The figure shows three views and two pictorial views of one solid part (mm, origin at its lowest corner). Answer the questions. A direction names the side the tool comes from. Coordinates: 2 decimals unless noted, no trailing zeros. Order: outer loops, then holes, each group sorted by start corner. A loop starts at its lowest first (then second) coordinate and runs counter-clockwise, first axis right, second up.
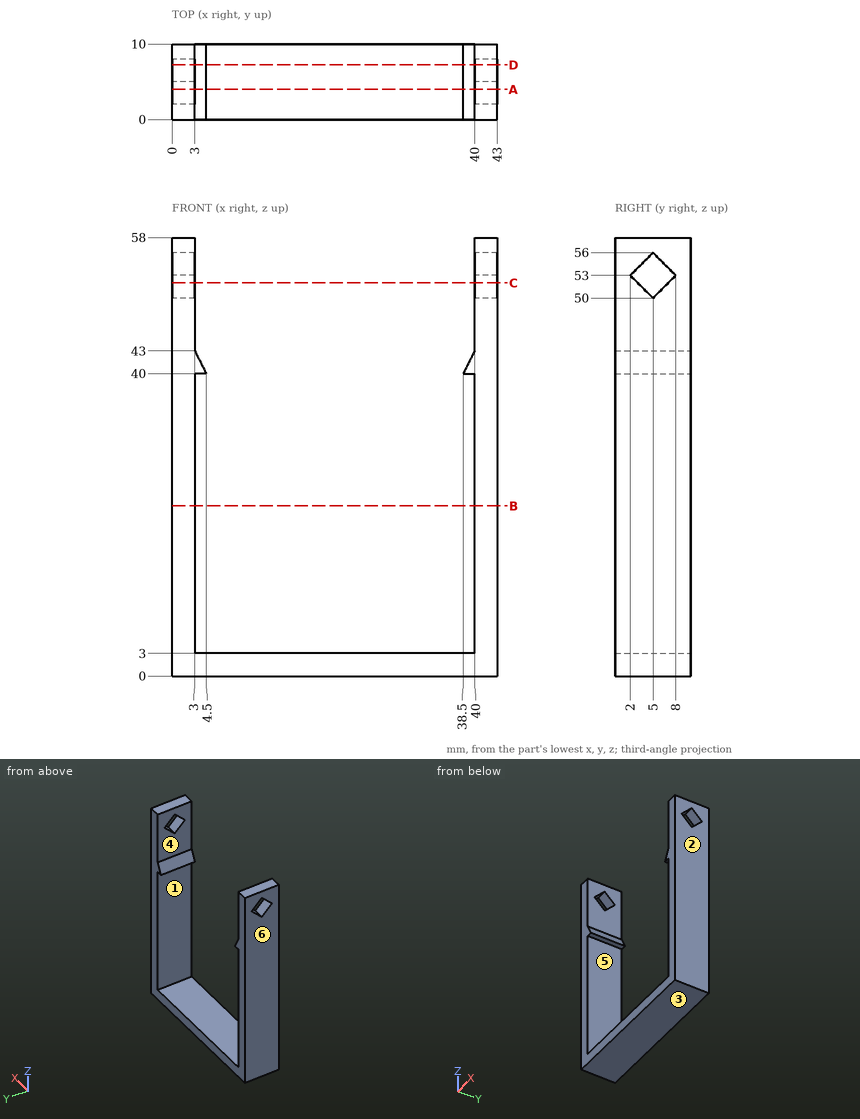
1) A cutting plane is placed at B-B, the plane z = 22.5. Write down the section's boundary in (x, y).
2) This flat-tipped pin is pushed along its axis until it touches: P1, Ø2, axis at x = 6, y = 2.5, coming from the +Z side. Where does it stop, or does it pass through?
3) For the marked faces 4, 5 and 6, determine the directions among +Z, -Z, +X, -X, +Y, -Y from which every point of the face is accessible in a straight line to the end or side of a thin tool.
4) The mould has two halves that part along Z. Classify the marked faces 1, 2 and 3: released by +Z, released by -Z, zero draft, split by the parting line, or undercut.
5) Straight lines are drawn through the part: probe 1 along X at (y, z) = (2.25, 3.5); probe 2 along Z at (x, y) = (12.5, 3.75); probe 3 along Z at (x, y) = (3.5, 9). For each, find the intervals that lie inside material, in ascending order.
6) A cutting plane is placed at C-C, the plane z = 52. Write down the section's boundary in (x, y).
7) A cutting plane is placed at D-D, the plane y = 7.25. Write down the section's boundary in (x, z).
8) A cutting plane is placed at A-A, the plane y = 4. Write down the section's boundary in (x, z).
Working result:
1. outline: (0, 0) - (3, 0) - (3, 10) - (0, 10) - close; (40, 0) - (43, 0) - (43, 10) - (40, 10) - close
2. P1: stops at z = 3
3. face 4: +Z, +Y, -Y
3. face 5: +Y, -Y
3. face 6: +Z, -Z, -X, +Y, -Y
4. face 1: undercut
4. face 2: zero draft
4. face 3: released by -Z
5. probe 1: x = 0 to 3, 40 to 43
5. probe 2: z = 0 to 3
5. probe 3: z = 0 to 3, 40 to 42
6. outline: (0, 0) - (3, 0) - (3, 3) - (0, 3) - close; (0, 7) - (3, 7) - (3, 10) - (0, 10) - close; (40, 0) - (43, 0) - (43, 3) - (40, 3) - close; (40, 7) - (43, 7) - (43, 10) - (40, 10) - close
7. outline: (0, 0) - (43, 0) - (43, 52.25) - (40, 52.25) - (40, 43) - (38.5, 40) - (40, 40) - (40, 3) - (3, 3) - (3, 40) - (4.5, 40) - (3, 43) - (3, 52.25) - (0, 52.25) - close; (0, 53.75) - (3, 53.75) - (3, 58) - (0, 58) - close; (40, 53.75) - (43, 53.75) - (43, 58) - (40, 58) - close
8. outline: (0, 0) - (43, 0) - (43, 51) - (40, 51) - (40, 43) - (38.5, 40) - (40, 40) - (40, 3) - (3, 3) - (3, 40) - (4.5, 40) - (3, 43) - (3, 51) - (0, 51) - close; (0, 55) - (3, 55) - (3, 58) - (0, 58) - close; (40, 55) - (43, 55) - (43, 58) - (40, 58) - close
